Source: CAD feature listing. Evaluate the final solid. Frame: model axes, mm. Round coordinates to 2 decimals unless told otherwise and drop trailing zeros. Loops run counter-clockwise (first coordinate to the right, second up) from the corner with the lowest first, then second, coordinate; pieces in that order, holes last. Notation, with made-up numbers: M 37,21 L 86,21 A15 cw 86,41 Z; hole C -4.75,-1 d10. An arc over 180 degrees is marked long. Answer as a JSON object with one key per item and string values.
from build123d import *

# Parameters (mm, degrees)
SKETCH1_W                = 160
SKETCH1_H                = 100
BOSS_EXTRUDE1_DEPTH      = 3
M3_CLEARANCE_HOLE1_D     = 3.4
CUT_EXTRUDE1_REACH       = 96.387
SKETCH8_W                = 20
SKETCH8_H                = 10
M3_CLEARANCE_HOLE3_D     = 3.4
M3_CLEARANCE_HOLE4_D     = 3.4
M3_CLEARANCE_HOLE4_DEPTH = 3
FILLET1_R                = 5
FILLET2_R                = 2


with BuildPart() as part:
    # Sketch1 → Boss-Extrude1 (new body)
    with BuildSketch(Plane(origin=(0, 0, 0), x_dir=(1, 0, 0), z_dir=(0, 1, 0))):
        Rectangle(SKETCH1_W, SKETCH1_H)
    extrude(amount=BOSS_EXTRUDE1_DEPTH)

    # M3 Clearance Hole1 (through all)
    with Locations(Plane(origin=(-68, 3, -14.9), x_dir=(0, 0, 1), z_dir=(0, 1, 0))):
        with Locations((0, 0), (0, 24), (29.8, 0), (29.8, 24), (0, 136), (0, 112), (29.8, 112), (29.8, 136)):
            Hole(M3_CLEARANCE_HOLE1_D / 2)

    # Sketch8 → Cut-Extrude1 (cut, up to next)
    with BuildSketch(Plane(origin=(0, 3, 0), x_dir=(1, 0, 0), z_dir=(0, 1, 0)), mode=Mode.PRIVATE) as cut_extrude1_sk1:
        with Locations((1, -35)):
            Rectangle(SKETCH8_W, SKETCH8_H)
    cut_extrude1_tool1 = extrude(cut_extrude1_sk1.sketch, amount=-CUT_EXTRUDE1_REACH, mode=Mode.PRIVATE) & part.part
    # Sketch8 → Cut-Extrude1 (cut, up to next)
    with BuildSketch(Plane(origin=(0, 3, 0), x_dir=(1, 0, 0), z_dir=(0, 1, 0)), mode=Mode.PRIVATE) as cut_extrude1_sk2:
        with Locations((1, 35)):
            Rectangle(SKETCH8_W, SKETCH8_H)
    cut_extrude1_tool2 = extrude(cut_extrude1_sk2.sketch, amount=-CUT_EXTRUDE1_REACH, mode=Mode.PRIVATE) & part.part
    add(cut_extrude1_tool1.solids().sort_by_distance((1, 3, 35))[0], mode=Mode.SUBTRACT)
    add(cut_extrude1_tool2.solids().sort_by_distance((1, 3, -35))[0], mode=Mode.SUBTRACT)

    # M3 Clearance Hole3 (through all)
    with Locations(Plane(origin=(0, 3, 0), x_dir=(1, 0, 0), z_dir=(0, 1, 0))):
        with Locations((-5.121033698, 7.476676114), (-5.143854766, -7.584150602)):
            Hole(M3_CLEARANCE_HOLE3_D / 2)

    # M3 Clearance Hole4
    with Locations(Plane(origin=(0, 3, 0), x_dir=(1, 0, 0), z_dir=(0, 1, 0))):
        with Locations((-62, 35), (-62, 42), (-69, 35), (-62, 28), (-55, 35), (-62, -42), (-69, -35), (-62, -28), (-55, -35), (-62, -35), (-17.29999936, -19.19999912), (39.0999996, 4.1), (-5.121033698, 7.476676114), (-5.143854766, -7.584150602), (62, -35), (69, -35), (62, -42), (55, -35), (62, -28), (69, 35), (62, 35), (62, 42), (55, 35), (62, 28)):
            Hole(M3_CLEARANCE_HOLE4_D / 2, depth=M3_CLEARANCE_HOLE4_DEPTH)

    # Fillet1
    fillet1_edges = [part.edges().sort_by_distance(p)[0] for p in [
        (80, 1.5, 50),
        (-80, 1.5, 50),
        (-80, 1.5, -50),
        (80, 1.5, -50),
    ]]
    fillet(fillet1_edges, radius=FILLET1_R)

    # Fillet2
    fillet2_edges = [part.edges().sort_by_distance(p)[0] for p in [
        (-9, 1.5, 40),
        (-9, 1.5, 30),
        (11, 1.5, 30),
        (11, 1.5, 40),
        (-9, 1.5, -30),
        (-9, 1.5, -40),
        (11, 1.5, -40),
        (11, 1.5, -30),
    ]]
    fillet(fillet2_edges, radius=FILLET2_R)


solid = part.part
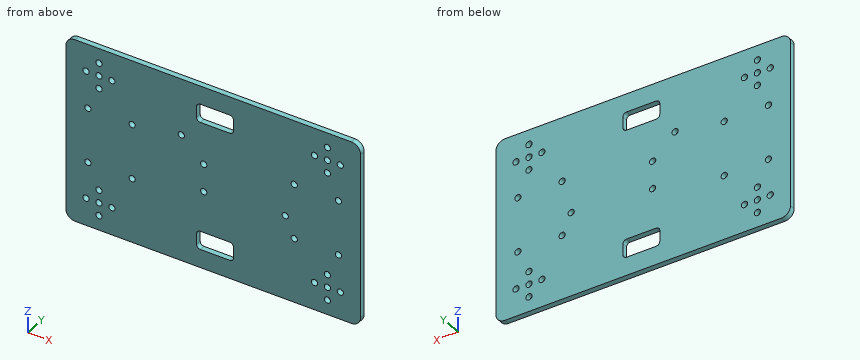
Item 1: Contact query for a flat-ended pin moving along its axis: pin 1 Ø3 at (x, z) = (-5.14, 7.58) entering from +Y. Output: stop coordinate, or through.
Answer sheet:
{"pin 1": "passes through"}
Item 2: Section D-D on y = 1. Give the number of separate pieces and of enclosed holes in the cut face, then the cut area to 3 significant figures.
Answer sheet:
{"separate pieces": "1", "enclosed holes": "34", "area": "15,300 mm²"}
Item 3: Section C-C on z = -42. Return the cut outline in (x, y).
Answer sheet:
{"outline": "M -80,0 L -63.7,0 L -63.7,3 L -80,3 Z; M -60.3,0 L 60.3,0 L 60.3,3 L -60.3,3 Z; M 63.7,0 L 80,0 L 80,3 L 63.7,3 Z"}
Item 4: Section A-A on x = -62. Return the cut outline in (y, z), then the cut area to 3 significant figures.
Answer sheet:
{"outline": "M 0,-50 L 3,-50 L 3,-43.7 L 0,-43.7 Z; M 0,-40.3 L 3,-40.3 L 3,-36.7 L 0,-36.7 Z; M 0,-33.3 L 3,-33.3 L 3,-29.7 L 0,-29.7 Z; M 0,-26.3 L 3,-26.3 L 3,26.3 L 0,26.3 Z; M 0,29.7 L 3,29.7 L 3,33.3 L 0,33.3 Z; M 0,36.7 L 3,36.7 L 3,40.3 L 0,40.3 Z; M 0,43.7 L 3,43.7 L 3,50 L 0,50 Z", "area": "239 mm²"}
Item 5: Line query: probe 1 along Z at (x, y) = (-5, 2.1); probe 2 along Z at (x, y) = (-55, 1.55); probe 3 along Z at (x, y) = (-1, 2.3). Output: solid intervals per line, ascending. Write a range as from..to.
Answer sheet:
{"probe 1": "z = -50..-40, -30..-9.17, -5.78..5.89, 9.28..30, 40..50", "probe 2": "z = -50..-36.7, -33.3..33.3, 36.7..50", "probe 3": "z = -50..-40, -30..30, 40..50"}
Item 6: Section B-B on x = 44. Return the cut outline in (y, z), then the cut area to 3 significant figures.
Answer sheet:
{"outline": "M 0,-50 L 3,-50 L 3,-16.6 L 0,-16.6 Z; M 0,-13.2 L 3,-13.2 L 3,13.2 L 0,13.2 Z; M 0,16.6 L 3,16.6 L 3,50 L 0,50 Z", "area": "280 mm²"}
